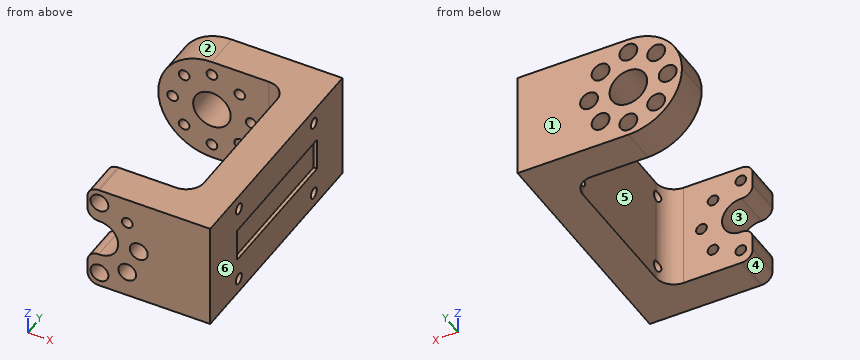
```python
from build123d import *

# Parameters (mm, degrees)
F1_DEPTH  = 30
F2_R      = 14.99999
F3_R      = 5.25
F4_DEPTH  = 100
F5_R      = 2.5
F6_DEPTH  = 7
F7_DEPTH  = 7
F8_R      = 1.5
F9_DEPTH  = 100
F10_R     = 2.5
F10_R_2   = 1.5
F11_DEPTH = 7
F12_W     = 19.7517806664
F12_H     = 36.5692139603
F13_DEPTH = 25
F14_R     = 3
F15_R     = 5
F16_R     = 1.5
F17_DEPTH = 25
F18_W     = 40.5211038888
F18_H     = 9.174589999
F19_DEPTH = 1


# Not quite as in the source:
# - a fillet or chamfer is up to 0.001 mm smaller than in the source, because OpenCascade refuses the exact size


with BuildPart() as f1:
    # F0 (on Top) → F1 (new body)
    with BuildSketch(Plane.XY):
        Polygon((26.5140141845, 39.809118801), (-19.4859858155, 39.809118801), (-19.4859858155, 29.809118801), (16.5140141845, 29.809118801), (16.5140141845, -17.190881199), (-19.4859858155, -17.190881199), (-19.4859858155, -27.190881199), (26.5140141845, -27.190881199), align=None)
    extrude(amount=F1_DEPTH)

    # F2 (radius 15 in the source; OpenCascade refuses exactly that, so slightly less here)
    f2_edges = [f1.edges().sort_by_distance(p)[0] for p in [
        (-19.485986, 34.809119, 30),
        (-19.485986, 34.809119, 0),
        (-19.485986, -22.190881, 30),
        (-19.485986, -22.190881, 0),
    ]]
    fillet(f2_edges, radius=F2_R)

    # F3 (on face) → F4 (cut)
    with BuildSketch(Plane(origin=(0, 39.809118801, 0), x_dir=(-1, 0, 0), z_dir=(0, 1, 0))):
        with Locations((4.4859858155, 15)):
            Circle(F3_R)
    extrude(amount=-F4_DEPTH, mode=Mode.SUBTRACT)

    # F5 (on face) → F6 (cut)
    with BuildSketch(Plane(origin=(0, 39.809118801, 0), x_dir=(-1, 0, 0), z_dir=(0, 1, 0))):
        with Locations((4.4859858155, 26)):
            Circle(F5_R)
    extrude(amount=-F6_DEPTH, mode=Mode.SUBTRACT)

    # F5 (on face) → F7 (cut)
    with BuildSketch(Plane(origin=(0, 39.809118801, 0), x_dir=(-1, 0, 0), z_dir=(0, 1, 0))):
        with Locations((-3.2921887775, 22.7781745931)):
            Circle(F5_R)
        with Locations((-6.5140141845, 15)):
            Circle(F5_R)
        with Locations((-3.2921887775, 7.2218254069)):
            Circle(F5_R)
        with Locations((4.4859858155, 4)):
            Circle(F5_R)
        with Locations((12.2641604086, 7.2218254069)):
            Circle(F5_R)
        with Locations((15.4859858155, 15)):
            Circle(F5_R)
        with Locations((12.2641604086, 22.7781745931)):
            Circle(F5_R)
    extrude(amount=-F7_DEPTH, mode=Mode.SUBTRACT)

    # F8 (on face) → F9 (cut)
    with BuildSketch(Plane(origin=(0, 39.809118801, 0), x_dir=(-1, 0, 0), z_dir=(0, 1, 0))):
        with Locations((4.4859858155, 26)):
            Circle(F8_R)
        with Locations((12.2641604086, 22.7781745931)):
            Circle(F8_R)
        with Locations((15.4859858155, 15)):
            Circle(F8_R)
        with Locations((12.2641604086, 7.2218254069)):
            Circle(F8_R)
        with Locations((4.4859858155, 4)):
            Circle(F8_R)
        with Locations((-3.2921887775, 7.2218254069)):
            Circle(F8_R)
        with Locations((-6.5140141845, 15)):
            Circle(F8_R)
        with Locations((-3.2921887775, 22.7781745931)):
            Circle(F8_R)
    extrude(amount=-F9_DEPTH, mode=Mode.SUBTRACT)

    # F10 (on face) → F11 (cut)
    with BuildSketch(Plane.XZ.offset(27.190881199)):
        with Locations((-4.4859858155, 26)):
            Circle(F10_R)
        with Locations((-4.4859858155, 26)):
            Circle(F10_R_2, mode=Mode.SUBTRACT)
        with Locations((-12.2641604086, 22.7781745931)):
            Circle(F10_R)
        with Locations((-12.2641604086, 22.7781745931)):
            Circle(F10_R_2, mode=Mode.SUBTRACT)
        with Locations((-15.4859858155, 15)):
            Circle(F10_R)
        with Locations((-15.4859858155, 15)):
            Circle(F10_R_2, mode=Mode.SUBTRACT)
        with Locations((-12.2641604086, 7.2218254069)):
            Circle(F10_R)
        with Locations((-12.2641604086, 7.2218254069)):
            Circle(F10_R_2, mode=Mode.SUBTRACT)
        with Locations((-4.4859858155, 4)):
            Circle(F10_R)
        with Locations((-4.4859858155, 4)):
            Circle(F10_R_2, mode=Mode.SUBTRACT)
        with Locations((3.2921887775, 7.2218254069)):
            Circle(F10_R)
        with Locations((3.2921887775, 7.2218254069)):
            Circle(F10_R_2, mode=Mode.SUBTRACT)
        with Locations((6.5140141845, 15)):
            Circle(F10_R)
        with Locations((6.5140141845, 15)):
            Circle(F10_R_2, mode=Mode.SUBTRACT)
        with Locations((-4.4859858155, 26)):
            Circle(F10_R_2)
    extrude(amount=-F11_DEPTH, mode=Mode.SUBTRACT)

    # F12 (on face) → F13 (cut)
    with BuildSketch(Plane.XZ.offset(27.190881199)):
        with Locations((-17.6862510853, 15.8640302252)):
            Rectangle(F12_W, F12_H)
    extrude(amount=-F13_DEPTH, mode=Mode.SUBTRACT)

    # F14
    f14_edges = [f1.edges().sort_by_distance(p)[0] for p in [
        (-7.810361, -22.190881, 29.626982),
        (-7.810361, -22.190881, 0.373018),
        (-7.810361, -22.190881, 10.936623),
        (-7.810361, -22.190881, 19.063377),
    ]]
    fillet(f14_edges, radius=F14_R)

    # F15
    f15_edges = [f1.edges().sort_by_distance(p)[0] for p in [
        (16.514014, 29.809119, 15),
        (16.514014, -17.190881, 15),
    ]]
    fillet(f15_edges, radius=F15_R)

    # F16 (on face) → F17 (cut)
    with BuildSketch(Plane.YZ.offset(26.5140141845)):
        with Locations((-12.690881199, 26)):
            Circle(F16_R)
        with Locations((-12.690881199, 4)):
            Circle(F16_R)
        with Locations((25.309118801, 4)):
            Circle(F16_R)
        with Locations((25.309118801, 26)):
            Circle(F16_R)
    extrude(amount=-F17_DEPTH, mode=Mode.SUBTRACT)

    # F18 (on face) → F19 (cut)
    with BuildSketch(Plane.YZ.offset(26.5140141845)):
        with Locations((6.6909566522, 15.1345017366)):
            Rectangle(F18_W, F18_H)
    extrude(amount=-F19_DEPTH, mode=Mode.SUBTRACT)


solid = f1.part
```
Here's how the part is built. I have some questions about the finished solid (model axes, mm). Face numbers are marked on the shaded views. A direction names the side the tool comes from. Coordinates: 2 decimals unless noted, no trailing zeros. Loops run counter-clockwise (first coordinate to the right, second up) from the corner with the lowest first, then second, coordinate; pieces in that order, holes last. Notation, with made-up numbers: (-4.75, -34.5) - (10.25, -34.5) arc R5 cw to (10.25, -26.5) - close; hole circle Ø6 at (-24.5, 31.25). An arc over 180 degrees is marked (long way). Return JSON: item names as keys, results as strings. Group by question number.
Item 1: If we section it at B-B on z = 19: Write out the boundary of the cut face in (x, y).
Item 2: I need wall thicknesses on line 1 (Y direction, x = 20, z = 4); line 2 (Y direction, x = 9.5, z = 24.5); line 3 (Y direction, x = 1, z = 8). Which ranges of each line are inside material? Lowest first, please. Write a range as from..to.
Item 3: Will these pins go through, and if not, where does the flat tip stop? P1, Ø4, axis at x = 6.51, z = 15, coming from the +Y side; P2, Ø1.1, axis at y = -23.5, z = 26, coming from the -X side; P3, Ø3, axis at y = -3.5, z = 11, coming from the -X side.
Item 4: On a 3-axis mill with a long thin cutter (end or side, diameter ignored), from which of +Z, -Z, +X, -X, +Y, -Y can I reach the whole of each face in a straight line? I mean the marked faces 4, 5 and 6. Say none if no direction works.
Item 5: If we section it at A-A on y = 26: Write out the boundary of the cut face in (x, z), and give its area (3 significant figures).
Item 6: We'd pull the mould along Z, two halves only. Please class the marked faces 1, 2 and 3: +Z half, -Z half, draft (parallel to the pull), parting line (faces both ways), or undercut.
Item 7: If we section it at C-C on z = 26: State how many separate pieces and enclosed holes the cut face has, and give its area (3 significant figures).
Calculated:
{
 "1": {"outline": "(-18.94, 29.81) - (-7.89, 29.81) - (-7.89, 39.81) - (-18.94, 39.81) - close; (-1.09, -27.19) - (26.51, -27.19) - (26.51, -13.57) - (25.51, -13.57) - (25.51, 26.95) - (26.51, 26.95) - (26.51, 39.81) - (-1.09, 39.81) - (-1.09, 29.81) - (11.51, 29.81) arc R5 cw to (16.51, 24.81) - (16.51, -12.19) arc R5 cw to (11.51, -17.19) - (-1.09, -17.19) - close"},
 "2": {"line 1": "y = -27.19..-14.19, -11.19..23.81, 26.81..39.81", "line 2": "y = -27.19..-17.19, 29.81..39.81", "line 3": "y = -20.19..-17.19, 29.81..32.81"},
 "3": {"P1": "stops at y = 32.81", "P2": "stops at x = -7.81", "P3": "stops at x = 16.51"},
 "4": {"face 4": "-Z, -X, -Y", "face 5": "+Z, -Z, -X", "face 6": "+Z, -Z, +X, +Y, -Y"},
 "5": {"outline": "(16.37, 0) - (26.51, 0) - (26.51, 2.67) - (16.37, 2.67) - close; (16.37, 5.33) - (26.51, 5.33) - (26.51, 10.55) - (25.51, 10.55) - (25.51, 19.72) - (26.51, 19.72) - (26.51, 24.67) - (16.37, 24.67) - close; (16.37, 27.33) - (26.51, 27.33) - (26.51, 30) - (16.37, 30) - close", "area": "241 mm^2"},
 "6": {"face 1": "draft", "face 2": "+Z half", "face 3": "undercut"},
 "7": {"separate pieces": "5", "enclosed holes": "0", "area": "1,090 mm^2"}
}
